```python
from build123d import *

# Parameters (mm, degrees)
SKETCH1_R           = 4.3688
SKETCH1_R_2         = 3.048
BOSS_EXTRUDE1_DEPTH = 6.35


with BuildPart() as part:
    # Sketch1 → Boss-Extrude1 (new body)
    with BuildSketch(Plane(origin=(0, 0, 0), x_dir=(1, 0, 0), z_dir=(0, 1, 0))):
        Polygon((152.4, 152.4), (77.73162, 152.4), (77.73162, -25.4), (-37.33419, -25.4), (-37.33419, -152.4), (152.4, -152.4), (152.4, 48.26), (97.79, 48.26), (97.79, 118.11), (152.4, 118.11), align=None)
        with Locations((-13.91158, -132.334)):
            Circle(SKETCH1_R, mode=Mode.SUBTRACT)
        with Locations((-13.91158, -62.484)):
            Circle(SKETCH1_R, mode=Mode.SUBTRACT)
        with Locations((94.03842, -132.334)):
            Circle(SKETCH1_R, mode=Mode.SUBTRACT)
        with Locations((94.03842, -62.484)):
            Circle(SKETCH1_R, mode=Mode.SUBTRACT)
        with Locations((87.68842, 27.94)):
            Circle(SKETCH1_R_2, mode=Mode.SUBTRACT)
        with Locations((142.367, 27.94)):
            Circle(SKETCH1_R_2, mode=Mode.SUBTRACT)
        with Locations((87.68842, 138.43)):
            Circle(SKETCH1_R_2, mode=Mode.SUBTRACT)
        with Locations((142.367, 138.43)):
            Circle(SKETCH1_R_2, mode=Mode.SUBTRACT)
    extrude(amount=BOSS_EXTRUDE1_DEPTH)


solid = part.part
```
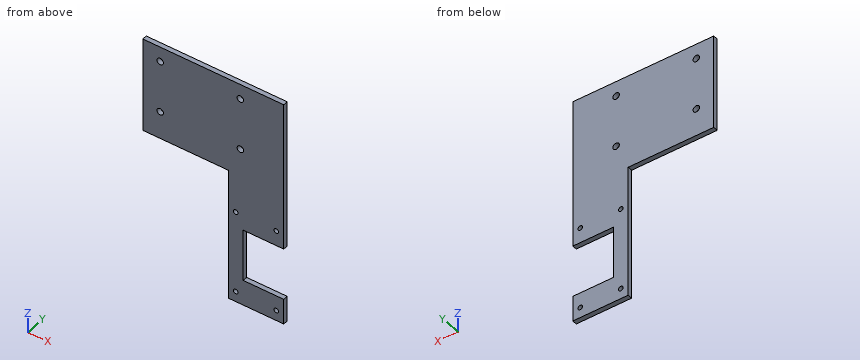
CAD build for the part. Positions are in the model's coordinates, mm. Round coordinates to 2 decimals unless told otherwise and drop trailing zeros. Order: outer loops, then holes, each group sorted by start corner. A loop starts at its lowest first (then second) coordinate and runs counter-clockwise, first axis right, second up. Notation, with made-up numbers: (40, 10) -> (65, 10) arc R32 cw to (65, 42) -> close; hole circle Ø11 at (-10, 84). An arc over 180 degrees is marked (long way). Write item = value, one per line.
(1) Cut at C-C (x = 51.5). Write the cut outline in (y, z).
Answers follow:
outline = (0, 25.4) -> (6.35, 25.4) -> (6.35, 152.4) -> (0, 152.4) -> close
(2) Flat gauge pins, fed straight in: P1, Ø3, axis at y = 0.5, z = -102, coming from the -X side; P2, Ø8, axis at x = -13.91, z = 132.33, coming from the +Y side (3 decimals); P3, Ø3, axis at x = 8.5, y = 1.5, coming from the -Z side; P4, Ø1.9, axis at y = 3.5, z = -83.5, coming from the +X side. Where does each tip first touch, or does it go through?
Answers follow:
P1 = 77.73
P2 = through
P3 = 25.4
P4 = 97.79
(3) Cut at A-A (z = -27.94). Write the cut outline in (x, y) (3 decimals).
Answers follow:
outline = (77.732, 0) -> (84.64, 0) -> (84.64, 6.35) -> (77.732, 6.35) -> close; (90.736, 0) -> (139.319, 0) -> (139.319, 6.35) -> (90.736, 6.35) -> close; (145.415, 0) -> (152.4, 0) -> (152.4, 6.35) -> (145.415, 6.35) -> close
(4) Cut at B-B (y = 4.75). State how many separate pieces and enclosed holes the cut face has, plus the area to 3 significant figures.
Answers follow:
separate_pieces = 1
enclosed_holes = 8
area = 33,200 mm²
(5) Drill centre lines: L1, parallel to Z at x = 93.5, y = 3.75; L2, parallel to Z at x = -14, y = 4.5; L3, parallel to X at y = 2.25, z = -27.94 (3 decimals). Where is each one in solid material? Low to high.
Answers follow:
L1 = -152.4 to 58.15, 66.82 to 128, 136.67 to 152.4
L2 = 25.4 to 58.12, 66.85 to 127.97, 136.7 to 152.4
L3 = 77.732 to 84.64, 90.736 to 139.319, 145.415 to 152.4
